Source: CAD feature listing. Evaluate the final solid. Frame: model axes, mm. Coordinates: 2 decimals unless noted, no trailing zeros. Loops run counter-clockwise (first coordinate to the right, second up) from the corner with the lowest first, then second, coordinate; pieces in that order, holes last. Notation, with made-up numbers: (22.5, 17.5) -> (30.5, 17.5) arc R25 ccw to (30.5, 56.5) -> close; hole circle Ø4 at (37, 5). An arc over 180 degrees is marked (long way). Answer as CSV lines item,"result".
from build123d import *

# Parameters (mm, degrees)
SKETCH_R     = 5
PAD_DEPTH    = 3
PAD001_DEPTH = 0.5


with BuildPart() as part:
    # Sketch → Pad (new body)
    with BuildSketch(Plane.XY):
        Circle(SKETCH_R)
    extrude(amount=PAD_DEPTH)

    # Sketch001 → Pad001 (join)
    with BuildSketch(Plane.XY):
        with BuildLine():
            Line((4.974937, 0.5), (5.974937, 0.5))
            Line((5.974937, 0.5), (5.974937, -0.5))
            Line((5.974937, -0.5), (4.974937, -0.5))
            ThreePointArc((4.974937, -0.5), (5, 0), (4.974937, 0.5))
        make_face()
    extrude(amount=PAD001_DEPTH)


solid = part.part
(1) Cut plane B-B (x = 5.25). Return the cut outline in (y, z), then the cut area to 3 significant figures.
Computed values:
outline,"(-0.5, 0) -> (0.5, 0) -> (0.5, 0.5) -> (-0.5, 0.5) -> close"
area,"0.500 mm^2"
(2) Cut plane D-D (z = 2.2). Return the cut outline in (x, y), then the cut area to 3 significant figures.
Computed values:
outline,"circle Ø10 at (0, 0)"
area,"78.5 mm^2"
(3) Material intervals for L1, parallel to X at y = 0, z = 2.65; L2, parallel to X at y = -1, z = 0.4, sorted ascending. Write a range as [from, to].
Computed values:
L1,"[-5, 5]"
L2,"[-4.9, 4.9]"
(4) Cut plane A-A (y = 0). Return the cut outline in (x, z), then the cut area to 3 significant figures.
Computed values:
outline,"(-5, 0) -> (5.97, 0) -> (5.97, 0.5) -> (5, 0.5) -> (5, 3) -> (-5, 3) -> close"
area,"30.5 mm^2"
(5) Cut plane C-C (z = 0.3). Return the cut outline in (x, y), then the cut area to 3 significant figures.
Computed values:
outline,"(4.97, -0.5) -> (5.97, -0.5) -> (5.97, 0.5) -> (4.97, 0.5) arc R5 ccw (long way) to start"
area,"79.5 mm^2"
(6) Pin query (flat end, axial travel): pin 1 Ø1.5 at (x, z) = (-1, 2) entering from -Y; pin 2 Ø1.5 at (x, z) = (0.5, 1.5) entering from +Y; pin 3 Ø1.5 at (y, z) = (-3.5, 1) entering from +X; pin 4 Ø1 at (y, z) = (-3, 1.5) entering from -X. Return the tip coordinate at first contact, or that it passes through.
Computed values:
pin 1,"y = -4.99"
pin 2,"y = 5"
pin 3,"x = 4.18"
pin 4,"x = -4.33"
